Verification items for this drawing (mm, ordinates from the low corner). A direction names the side the tool comes from. Round coordinates to 2 decimals unless told otherwise and drop trailing zeros. Loops run counter-clockwise (first coordinate to the right, second up) from the corner with the lowest first, then second, coordinate; pieces in that order, holes last. Notation, with made-up numbers: M 61.5,-1 L 92.5,-1 A28 cw 92.5,24 Z; hole C -5.75,78 d6. An arc over 180 degrees is marked long. One line per item, written item: value.
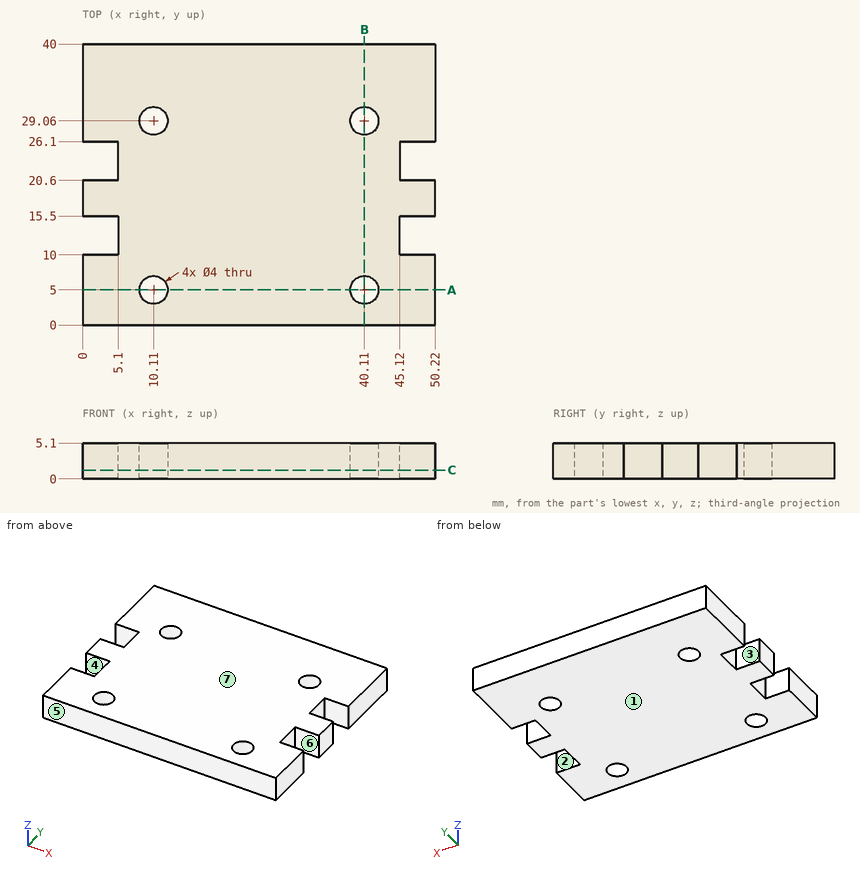
(1) Mould release check, pull along Y, two halves, no side actions. Record for the marked faces 4, 5, 6 and 7: +Y half, -Y half, draft (parallel to the pull), parting line (faces both ways), or undercut.
Completed:
face 4: undercut
face 5: -Y half
face 6: undercut
face 7: draft
(2) Thickness scan on L1, parallel to Y at x = 10.11, z = 3.7; L2, parallel to Y at x = 2, z = 1.55; L3, parallel to X at y = 25, z = 2. Record the ranges inside material, lowest first. Write a range as from..to.
Completed:
L1: y = 0..3, 7..27.06, 31.06..40
L2: y = 0..10, 15.5..20.6, 26.1..40
L3: x = 5.1..45.12
(3) Sectioned sample at A-A on y = 5. Enter the section's corners in (x, z).
Completed:
outline: M 0,0 L 8.11,0 L 8.11,5.1 L 0,5.1 Z; M 12.11,0 L 38.11,0 L 38.11,5.1 L 12.11,5.1 Z; M 42.11,0 L 50.22,0 L 50.22,5.1 L 42.11,5.1 Z
(4) Sectioned sample at B-B on x = 40.11. Enter the section's corners in (y, z).
Completed:
outline: M 0,0 L 3,0 L 3,5.1 L 0,5.1 Z; M 7,0 L 27.06,0 L 27.06,5.1 L 7,5.1 Z; M 31.06,0 L 40,0 L 40,5.1 L 31.06,5.1 Z
(5) Depth check by flat-ended pin: pin 1 Ø1.5 at (y, z) = (13.5, 3.5) entering from -X. Enter the tip coordinate at first touch or a pass-through.
Completed:
pin 1: stops at x = 5.1
(6) Sectioned sample at C-C on z = 1.25. Enter the section's corners in (x, y).
Completed:
outline: M 0,0 L 50.22,0 L 50.22,10 L 45.12,10 L 45.12,15.5 L 50.22,15.5 L 50.22,20.6 L 45.12,20.6 L 45.12,26.1 L 50.22,26.1 L 50.22,40 L 0,40 L 0,26.1 L 5.1,26.1 L 5.1,20.6 L 0,20.6 L 0,15.5 L 5.1,15.5 L 5.1,10 L 0,10 Z; hole C 10.11,5 d4; hole C 10.11,29.06 d4; hole C 40.11,5 d4; hole C 40.11,29.06 d4
(7) Tool access check on the marked faces 1, 2 and 3. Record the directions out of +Z, -Z, +X, -X, +Y, -Y that give a thin tool (end or side, any length) a straight path to the whole face; none if there is none.
Completed:
face 1: -Z, +X, -X, +Y, -Y
face 2: +Z, -Z, +X
face 3: +Z, -Z, -X
